The listing builds one solid part. Answer for the finished solid, in the listing's coordinates (mm). A direction names the side the tool comes from. Give positions to 0.01 mm unless a question says otherwise; leave off trailing zeros. Loops run counter-clockwise (first coordinate to the right, second up) from the corner with the lowest first, then second, coordinate; pieces in that order, holes last.
Item 1: Section C-C, the plane x = 54 is taken. Give the vertices of the cut face in (y, z), and give its area (3 significant figures).
Item 2: Each of these flat-tipped pins is pushed along its axis until it touches: pin 1 Ø1.1 at (x, z) = (48.5, 14.5) entering from +Y; pin 2 Ø10 at (y, z) = (108.5, 19.5) entering from -X. Where does it stop, or does it pass through?
Item 3: Section D-D, the plane z = 20.25 is taken. Give the vertices of the cut face in (x, y), and give its area (3 significant figures).
Item 4: The mould has two halves that part along Z. Classify faces 3 (the face through (51.418, 110.058, 15.335)), 4 (the face through (14, 97.536, 14)), 5 (the face through (31, 48, 0)): pulls with the +Z half, pulls with the -Z half, needs draft (parallel to the pull), parting line crosses it, or undercut.
Item 5: A tool of negligible diameter and unlimited length cuts with its end or side. For faces 1 (the face through (31, 48, 27.94)), 2 (the face through (16.366, 110.058, 15.335)), from which of +Z, -Z, +X, -X, +Y, -Y can it reach the whole face along a straight path? Write none if from no direction.
Item 6: Section A-A, the plane z = 13.97 is taken. Give the vertices of the cut face in (x, y).
Item 7: Consider line 1 along X through (y, z) = (104.25, 13.97); line 2 along Y through (x, z) = (61.5, 12). Determine where each line is inside the solid, lowest interval first.
Item 8: Section B-B, the plane y = 102.5 is taken. Give the vertices of the cut face in (x, z) (3 decimals), and give its area (3 significant figures).
from build123d import *

# Parameters (mm, degrees)
SKETCH1_W           = 63.5
SKETCH1_H           = 27.94
BOSS_EXTRUDE1_DEPTH = 97.536
SKETCH2_R           = 2.54
SKETCH2_R_2         = 1.905
BOSS_EXTRUDE2_DEPTH = 25.4


with BuildPart() as part:
    # Sketch1 → Boss-Extrude1 (new body)
    with BuildSketch(Plane(origin=(0, 0, 0), x_dir=(1, 0, 0), z_dir=(0, 1, 0))):
        with Locations((31.75, -13.97)):
            Rectangle(SKETCH1_W, SKETCH1_H)
    extrude(amount=BOSS_EXTRUDE1_DEPTH)

    # Sketch2 → Boss-Extrude2 (add)
    # profile 1 of 2: a face of its own
    with BuildSketch(Plane(origin=(0, 97.536, 0), x_dir=(1, 0, 0), z_dir=(0, 1, 0))):
        with Locations(Location((14.224, -13.97, 0), (0, 0, 270))):
            Circle(SKETCH2_R)
        with Locations(Location((14.224, -13.97, 0), (0, 0, 270))):
            Circle(SKETCH2_R_2, mode=Mode.SUBTRACT)
    # profile 2 of 2: a face of its own
    with BuildSketch(Plane(origin=(0, 97.536, 0), x_dir=(1, 0, 0), z_dir=(0, 1, 0))):
        with Locations(Location((49.276, -13.97, 0), (0, 0, 270))):
            Circle(SKETCH2_R)
        with Locations(Location((49.276, -13.97, 0), (0, 0, 270))):
            Circle(SKETCH2_R_2, mode=Mode.SUBTRACT)
    extrude(amount=BOSS_EXTRUDE2_DEPTH)


solid = part.part
Worked answers:
1. outline: (0, 0) - (97.54, 0) - (97.54, 27.94) - (0, 27.94) - close
1. area: 2,730 mm2
2. pin 1: stops at y = 97.54
2. pin 2: stops at x = 11.74
3. outline: (0, 0) - (63.5, 0) - (63.5, 97.54) - (0, 97.54) - close
3. area: 6,190 mm2
4. face 3: parting line crosses it
4. face 4: undercut
4. face 5: pulls with the -Z half
5. face 1: +Z, +X, -X, +Y, -Y
5. face 2: +Y
6. outline: (0, 0) - (63.5, 0) - (63.5, 97.54) - (51.82, 97.54) - (51.82, 122.94) - (51.18, 122.94) - (51.18, 97.54) - (47.37, 97.54) - (47.37, 122.94) - (46.74, 122.94) - (46.74, 97.54) - (16.76, 97.54) - (16.76, 122.94) - (16.13, 122.94) - (16.13, 97.54) - (12.32, 97.54) - (12.32, 122.94) - (11.68, 122.94) - (11.68, 97.54) - (0, 97.54) - close
7. line 1: x = 11.68 to 12.32, 16.13 to 16.76, 46.74 to 47.37, 51.18 to 51.82
7. line 2: y = 0 to 97.54
8. outline: circle Ø5.08 at (14.224, 13.97); circle Ø5.08 at (49.276, 13.97); hole circle Ø3.81 at (14.224, 13.97); hole circle Ø3.81 at (49.276, 13.97)
8. area: 17.7 mm2
